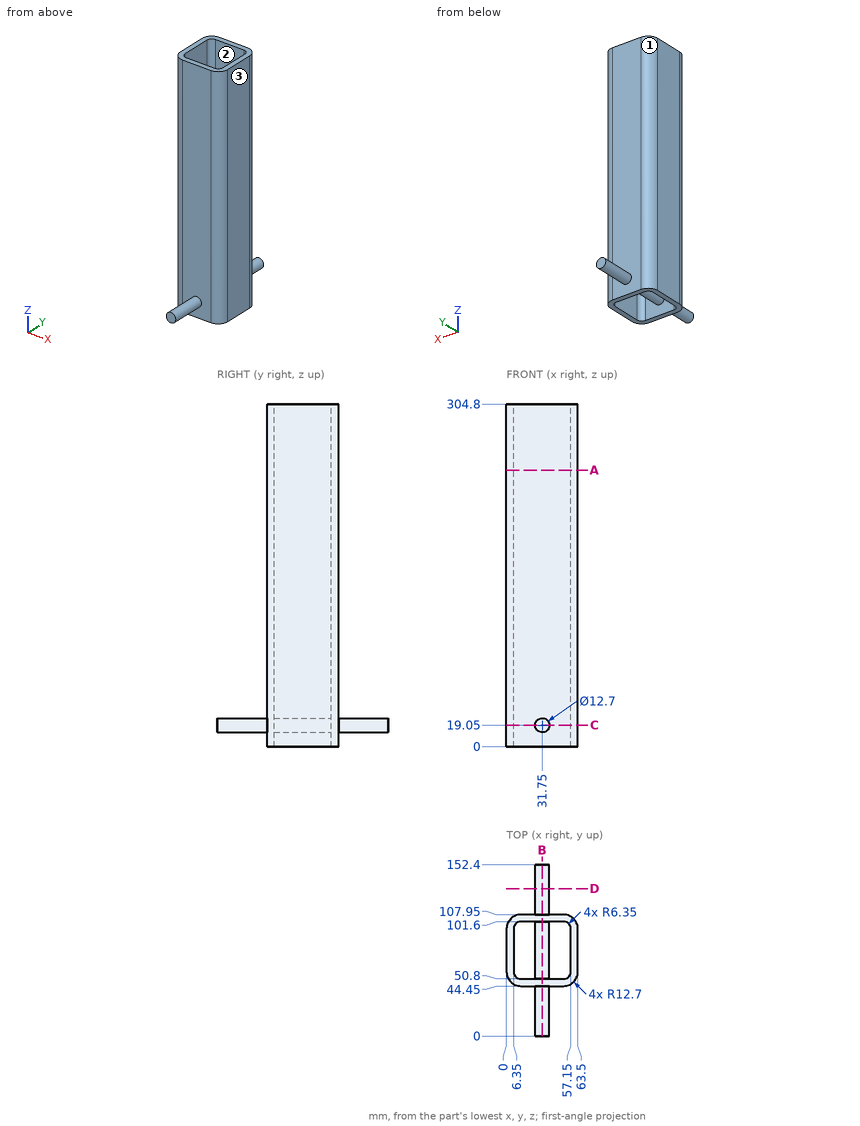
Can you work these out from the drawing? Everything is in mm from the part's minimum corner. Round coordinates to 2 decimals unless told otherwise and drop trailing zeros. Write each loop counter-clockwise with the first axis right and the second up, starting at its lowest first coordinate (ties: lowest second). Pieces come first, ordered by that corner, then holes.
1. Will these pins go through, and if not, where does the flat tip stop? pin 1 Ø10 at (y, z) = (101, 56.5) entering from +X; pin 2 Ø3 at (x, z) = (40.5, 31) entering from -Y; pin 3 Ø19 at (x, z) = (26.5, 225.5) entering from +Y.
2. Suppose I cut it at B-B (x = 31.75). List the corners of the cut face in (y, z) for me.
3. Suppose I cut it at A-A (z = 246). List the corners of the cut face in (x, y) for me, and give its area (3 significant figures).
4. I need wall thicknesses on L1, parallel to Y at x = 47.5, z = 74.5; L2, parallel to X at y = 80, z = 15; L3, parallel to X at y = 66.5, z = 81. Which ranges of each line are inside material? Lowest first, please.
5. Suppose I cut it at D-D (y = 131). List the corners of the cut face in (x, z) for me.
6. Suppose I cut it at C-C (z = 19.05). List the corners of the cut face in (x, y) for me, and give its area (3 significant figures).
7. If we mould it in two halves opening along Y, with no side actions, what happens to the marked faces 1, 2 and 3? For each: released by +Y, released by -Y, zero draft, split by the parting line, or undercut.
Answer sheet:
1. pin 1: stops at x = 63.48
1. pin 2: stops at y = 44.45
1. pin 3: stops at y = 107.95
2. outline: (0, 12.7) - (44.45, 12.7) - (44.45, 0) - (50.8, 0) - (50.8, 12.7) - (101.6, 12.7) - (101.6, 0) - (107.95, 0) - (107.95, 12.7) - (152.4, 12.7) - (152.4, 25.4) - (107.95, 25.4) - (107.95, 304.8) - (101.6, 304.8) - (101.6, 25.4) - (50.8, 25.4) - (50.8, 304.8) - (44.45, 304.8) - (44.45, 25.4) - (0, 25.4) - close
3. outline: (0, 57.15) arc R12.7 ccw to (12.7, 44.45) - (50.8, 44.45) arc R12.7 ccw to (63.5, 57.15) - (63.5, 95.25) arc R12.7 ccw to (50.8, 107.95) - (12.7, 107.95) arc R12.7 ccw to (0, 95.25) - close; hole (6.35, 57.15) arc R6.35 ccw to (12.7, 50.8) - (50.8, 50.8) arc R6.35 ccw to (57.15, 57.15) - (57.15, 95.25) arc R6.35 ccw to (50.8, 101.6) - (12.7, 101.6) arc R6.35 ccw to (6.35, 95.25) - close
3. area: 1,350 mm2
4. L1: y = 44.45 to 50.8, 101.6 to 107.95
4. L2: x = 0 to 6.35, 26.86 to 36.64, 57.15 to 63.5
4. L3: x = 0 to 6.35, 57.15 to 63.5
5. outline: circle Ø12.7 at (31.75, 19.05)
6. outline: (0, 57.15) arc R12.7 ccw to (12.7, 44.45) - (25.4, 44.45) - (25.4, 0) - (38.1, 0) - (38.1, 44.45) - (50.8, 44.45) arc R12.7 ccw to (63.5, 57.15) - (63.5, 95.25) arc R12.7 ccw to (50.8, 107.95) - (38.1, 107.95) - (38.1, 152.4) - (25.4, 152.4) - (25.4, 107.95) - (12.7, 107.95) arc R12.7 ccw to (0, 95.25) - close; hole (6.35, 57.15) arc R6.35 ccw to (12.7, 50.8) - (25.4, 50.8) - (25.4, 101.6) - (12.7, 101.6) arc R6.35 ccw to (6.35, 95.25) - close; hole (38.1, 50.8) - (50.8, 50.8) arc R6.35 ccw to (57.15, 57.15) - (57.15, 95.25) arc R6.35 ccw to (50.8, 101.6) - (38.1, 101.6) - close
6. area: 3,120 mm2
7. face 1: released by +Y
7. face 2: undercut
7. face 3: zero draft
